```python
from build123d import *

# Parameters (mm, degrees)
F0_W     = 40.219121
F0_H     = 42.154662
F1_DEPTH = 38.431481
F3_W     = 40.219121
F3_H     = 42.154662
F4_DEPTH = 282.206297


with BuildPart() as f1:
    # F0 (on Front) → F1 (new body)
    with BuildSketch(Plane.XZ):
        with Locations((20.109561, 31.930771)):
            Rectangle(F0_W, F0_H)
    extrude(amount=F1_DEPTH)

    # F3 (on face) → F4 (join)
    with BuildSketch(Plane.XZ.offset(38.431481)):
        with Locations((20.109561, 31.930771)):
            Rectangle(F3_W, F3_H)
        Polygon((37.252998, 38.319705), (29.511055, 20.913811), (12.105161, 28.655754), (19.847104, 46.061648), align=None, mode=Mode.SUBTRACT)
    extrude(amount=F4_DEPTH)


solid = f1.part
```
Design review of the part built by this model. Coordinates are the model's own, in mm. A direction names the side the tool comes from. Give positions to 0.01 mm unless a question says otherwise; leave off trailing zeros. Write each loop counter-clockwise with the first axis right and the second up, starting at its lowest first coordinate (ties: lowest second). Pieces come first, ordered by that corner, then holes. Notation, with made-up numbers: (-22.75, 7.25) -> (24.25, 7.25) arc R13 ccw to (24.25, 25.25) -> close; hole circle Ø7 at (0.25, 72.5). An arc over 180 degrees is marked (long way). Answer in a Markdown table with one row per item.
(1) Mouldability with a two-part tool opening along X and no side actions: class faces 1 (the flat face through (0, -158, 32)), 2 (the flat face through (15.922, -177.559, 37.237)), 3 (the flat face through (40.219, -158, 32)) as +X half, -X half, draft (parallel to the pull), parting line (faces both ways), or undercut.
Results:
| item | result |
|---|---|
| face 1 | -X half |
| face 2 | undercut |
| face 3 | +X half |
(2) Consider section A-A (y = -155.5). State the section outline as (x, z) points.
Results:
| item | result |
|---|---|
| outline | (0, 10.85) -> (40.22, 10.85) -> (40.22, 53.01) -> (0, 53.01) -> close; hole (12.11, 28.66) -> (29.51, 20.91) -> (37.25, 38.32) -> (19.85, 46.06) -> close |
(3) Consider section B-B (x = 15.5). State the section outline as (y, z) points, then the cut area to 3 significant figures.
Results:
| item | result |
|---|---|
| outline | (-320.64, 10.85) -> (0, 10.85) -> (0, 53.01) -> (-320.64, 53.01) -> (-320.64, 36.29) -> (-38.43, 36.29) -> (-38.43, 27.15) -> (-320.64, 27.15) -> close |
| area | 10,900 mm2 |
(4) To check wall thickness, follow probe 1 along Z at (x, y) = (27, -275.5); probe 2 along Z at (x, y) = (34, -160); probe 3 along X at (y, z) = (-300.5, 24). State the ranges of each line that lie inside material, in increasing order.
Results:
| item | result |
|---|---|
| probe 1 | 10.85 to 22.03, 42.88 to 53.01 |
| probe 2 | 10.85 to 31.01, 39.77 to 53.01 |
| probe 3 | 0 to 22.57, 30.88 to 40.22 |
(5) For faces 4 (the flat face through (20, -158, 10.853)), 5 (the flat face through (20.93, -177.56, 24.73)), list the 3-axis set-ups (+Z, -Z, +X, -X, +Y, -Y) from which the entire face can be reached by the end or side of a thin tool; tool diameter is ignored.
Results:
| item | result |
|---|---|
| face 4 | -Z, +X, -X, +Y, -Y |
| face 5 | -Y |
(6) Consider section C-C (z = 31.5). State the section outline as (x, y) points.
Results:
| item | result |
|---|---|
| outline | (0, -320.64) -> (13.37, -320.64) -> (13.37, -38.43) -> (34.22, -38.43) -> (34.22, -320.64) -> (40.22, -320.64) -> (40.22, 0) -> (0, 0) -> close |
